Drawing for the job (mm, zero at the part's lowest x, y, z). Give positions to 0.01 mm unless a question says otherwise; leave off trailing zeros. Write each loop counter-clockwise with the first axis right and the second up, starting at its lowest first coordinate (ties: lowest second). Pieces come first, ordered by that corner, then holes. Notation, with made-up numbers: M 51,69 L 94,69 A23 cw 94,94 Z; hole C 32.25,4 d9. An arc over 180 degrees is marked long. Write item = value, one per line. Start each with the question number.
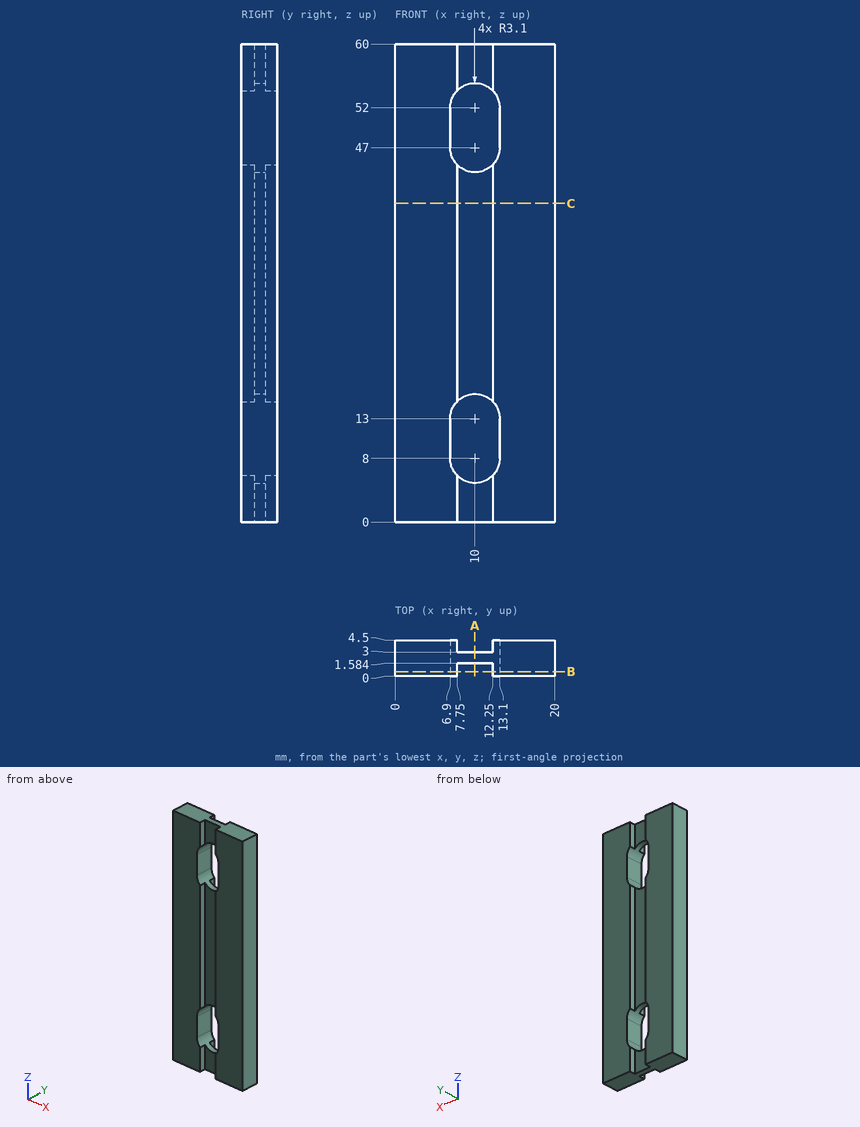
Q1. Slice it at B-B (y = 0.55). Give the cut face in (x, z).
Q2. Drop a flat-ended pin along its axis: P1, Ø3.5, axis at x = 10, z = 4.5, coming from the -Y side. Give the stop position or say it passes through.
Q3. Probe line 1 along X through (y, z) = (4.1, 23); line 2 along Y through (x, z) = (11, 19); line 3 along X through (y, z) = (4.2, 11.5). List the from-to ranges inside material, lowest first.
Q4. Slice it at C-C (z = 40). Give the cut face in (x, y), and give its area (3 significant figures).
Q5. Slice it at A-A (x = 10). Give the cut face in (y, z).
Working result:
q1.outline = M 0,0 L 7.75,0 L 7.75,5.87 A3.1 cw 6.9,8 L 6.9,13 A3.1 cw 7.75,15.13 L 7.75,44.87 A3.1 cw 6.9,47 L 6.9,52 A3.1 cw 7.75,54.13 L 7.75,60 L 0,60 Z; M 12.25,0 L 20,0 L 20,60 L 12.25,60 L 12.25,54.13 A3.1 cw 13.1,52 L 13.1,47 A3.1 cw 12.25,44.87 L 12.25,15.13 A3.1 cw 13.1,13 L 13.1,8 A3.1 cw 12.25,5.87 Z
q2.P1 = 1.58
q3.line_1 = 0 to 7.75, 12.25 to 20
q3.line_2 = 1.58 to 3
q3.line_3 = 0 to 6.9, 13.1 to 20
q4.outline = M 0,0 L 7.75,0 L 7.75,1.58 L 12.25,1.58 L 12.25,0 L 20,0 L 20,4.5 L 12.25,4.5 L 12.25,3 L 7.75,3 L 7.75,4.5 L 0,4.5 Z
q4.area = 76.1 mm2
q5.outline = M 1.58,0 L 3,0 L 3,4.9 L 1.58,4.9 Z; M 1.58,16.1 L 3,16.1 L 3,43.9 L 1.58,43.9 Z; M 1.58,55.1 L 3,55.1 L 3,60 L 1.58,60 Z
